Geometry: see drawing. Coordinates: mm, zero at the bounding-box minimum. Give positions to 0.01 mm unless a question says otherwise; leave off trailing zeros. Write each loop counter-clockwise with the first axis right and the second up, starting at its lowest first coordinate (ties: lowest second). Pieces come first, ordered by that corner, then holes. Notation, with made-up numbers: M 51,9.25 L 100,9.25 A27 cw 100,27.25 Z; hole C 6,74.25 d4. An arc over 180 degrees is marked long. Answer as a JSON object with one key per item and string values. Group by question number.
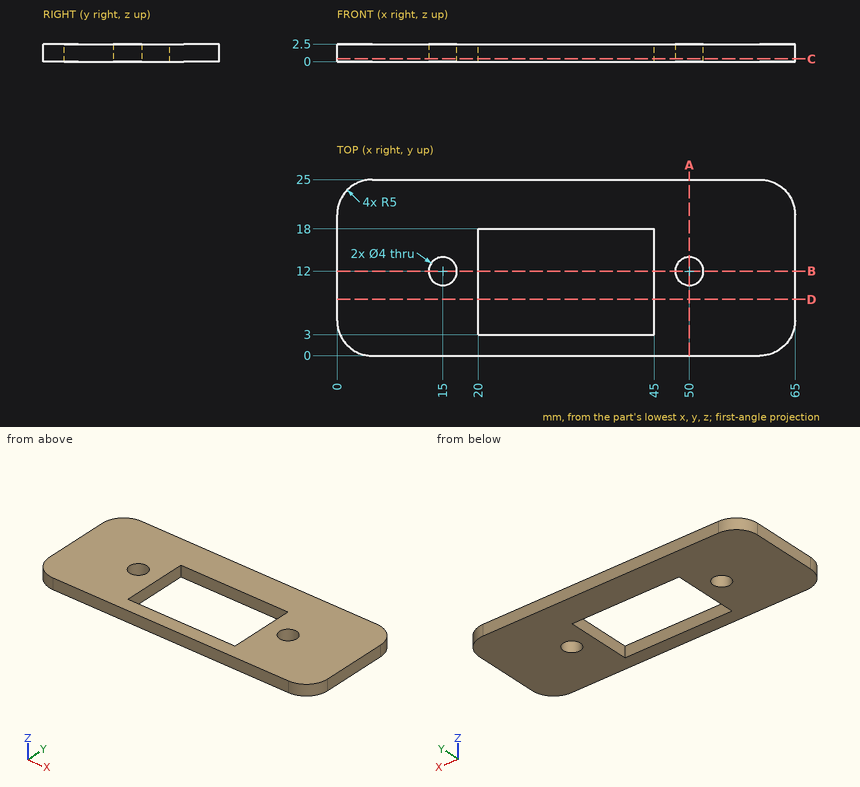
(1) Section A-A, the plane x = 50. Return loops of the section in (y, z), plus the area to 3 significant figures.
(2) Contact query for a flat-ended pin moving along its axis: pin 1 Ø1 at (x, y) = (22, 9.5) entering from +Z. Output: stop coordinate, or through.
(3) Section B-B, the plane y = 12. Return loops of the section in (x, z).
(4) Ray query, L1, parallel to Y at x = 50, z = 0.8; L2, parallel to X at y = 16, z = 1.2; L3, parallel to Y at x = 42.5, z = 1.65. Return the intervals inside material, ascending. Write a range as [from, to].
(5) Section C-C, the plane z = 0.4. Return loops of the section in (x, y).
(6) Section D-D, the plane y = 8. Return loops of the section in (x, z).
Reported:
{
 "1": {"outline": "M 0,0 L 10,0 L 10,2.5 L 0,2.5 Z; M 14,0 L 25,0 L 25,2.5 L 14,2.5 Z", "area": "52.5 mm2"},
 "2": {"pin 1": "passes through"},
 "3": {"outline": "M 0,0 L 13,0 L 13,2.5 L 0,2.5 Z; M 17,0 L 20,0 L 20,2.5 L 17,2.5 Z; M 45,0 L 48,0 L 48,2.5 L 45,2.5 Z; M 52,0 L 65,0 L 65,2.5 L 52,2.5 Z"},
 "4": {"L1": "y = [0, 10], [14, 25]", "L2": "x = [0, 20], [45, 65]", "L3": "y = [0, 3], [18, 25]"},
 "5": {"outline": "M 0,5 A5 ccw 5,0 L 60,0 A5 ccw 65,5 L 65,20 A5 ccw 60,25 L 5,25 A5 ccw 0,20 Z; hole C 15,12 d4; hole M 20,3 L 45,3 L 45,18 L 20,18 Z; hole C 50,12 d4"},
 "6": {"outline": "M 0,0 L 20,0 L 20,2.5 L 0,2.5 Z; M 45,0 L 65,0 L 65,2.5 L 45,2.5 Z"}
}
